Build history of the part. All positions in model axes, mm. A direction names the side the tool comes from. Give positions to 0.01 mm unless a question says otherwise; leave off trailing zeros. Write each loop counter-clockwise with the first axis right and the second up, starting at its lowest first coordinate (ties: lowest second). Pieces come first, ordered by that corner, then holes. Notation, with made-up numbers: M 17,84 L 58,84 A18 cw 58,96 Z; hole C 50.25,15.5 d7. An arc over 180 degrees is marked long. Return JSON: item names as keys, results as strings. Group by question number.
Q1. Pull direction Z, two halves, no side cores. Call faces 4 (the cylindrical face through (-1.08, 0.02, -4.88)), 5 (the flat face through (1, -5, -3.3)), 6 (the flat face through (2, 10, -5)): +Z half, -Z half, draft (parallel to the pull), parting line (faces both ways), or undercut.
Q2. Band-saw the part on B-B, the plane z = 0. Give the cut face in (x, y).
Q3. Band-saw the part on C-C, the plane y = -1. Give the cut face in (x, z), then the cut area to 3 significant figures.
Q4. Band-saw the part on D-D, the plane y = 3.5. Give the cut face in (x, z).
Q5. Wall check: probe 1 along X at (y, z) = (-7, -2.75); probe 2 along Z at (x, y) = (-1.25, 2.5); probe 3 along X at (y, z) = (5.25, -3.25). Give the ranges that are in metal, low to high.
Q6. Band-saw the part on A-A, the plane x = 0. Give the cut face in (y, z).
Q7. Flat gauge pins, fed straight in: pin 1 Ø2 at (x, y) = (-3.5, 2) entering from -Z; pin 2 Ø4 at (y, z) = (-4, 1.5) entering from +X; pin 3 Ø3 at (x, y) = (-1.5, -4.5) entering from +Z. Where does each tip first touch, or does it go through?
Q8. Tool access for faces 1 (the flat face through (-3.3, 5, -1)), 2 (the cylindrical face through (-1.08, -7.54, -4.88)), 3 (the conical face through (5.276, 3.921, -2.188)): list every direction of +Z, -Z, +X, -X, +Y, -Y with a clear straight run to the whole face (end or side of a thin tool).
from build123d import *

# Parameters (mm, degrees)
F0_W           = 5
F0_H           = 3
F3_D           = 6.5
F3_CBORE_D     = 10
F3_CBORE_DEPTH = 5
F4_R           = 5
F4_R_2         = 3.25
F5_DEPTH       = 5


with BuildPart() as f1:
    # F0 (on Top) → F1 (revolve)
    with BuildSketch(Plane.XY):
        Polygon((0, 1.5), (5, 1.5), (7.5, 10), (0, 10), align=None)
        Polygon((0, -10), (7.5, -10), (5, -1.5), (0, -1.5), align=None)
        with Locations((2.5, 0)):
            Rectangle(F0_W, F0_H)
    revolve(axis=Axis((0, 0, 0), (0, -1, 0)))

    # F3 (through all)
    with Locations(Plane(origin=(0, 10, 0), x_dir=(-1, 0, 0), z_dir=(0, 1, 0))):
        with Locations((0, 0)):
            CounterBoreHole(F3_D / 2, F3_CBORE_D / 2, F3_CBORE_DEPTH)

    # F4 (on face) → F5 (cut)
    with BuildSketch(Plane.XZ.offset(10)):
        Circle(F4_R)
        Circle(F4_R_2, mode=Mode.SUBTRACT)
    extrude(amount=-F5_DEPTH, mode=Mode.SUBTRACT)


solid = f1.part
From the geometry:
{
 "1": {"face 4": "parting line", "face 5": "undercut", "face 6": "draft"},
 "2": {"outline": "M -7.5,-10 L -5,-10 L -5,-5 L -3.25,-5 L -3.25,5 L -5,5 L -5,10 L -7.5,10 L -5,1.5 L -5,-1.5 Z; M 3.25,-5 L 5,-5 L 5,-10 L 7.5,-10 L 5,-1.5 L 5,1.5 L 7.5,10 L 5,10 L 5,5 L 3.25,5 Z"},
 "3": {"outline": "C 0,0 d10; hole C 0,0 d6.5", "area": "45.4 mm^2"},
 "4": {"outline": "C 0,0 d11.18; hole C 0,0 d6.5"},
 "5": {"probe 1": "x = -6.02 to -4.18, 4.18 to 6.02", "probe 2": "z = -5.14 to -3, 3 to 5.14", "probe 3": "x = -5.17 to -3.8, 3.8 to 5.17"},
 "6": {"outline": "M -10,-7.5 L -1.5,-5 L 1.5,-5 L 10,-7.5 L 10,-5 L 5,-5 L 5,-3.25 L -5,-3.25 L -5,-5 L -10,-5 Z; M -10,5 L -5,5 L -5,3.25 L 5,3.25 L 5,5 L 10,5 L 10,7.5 L 1.5,5 L -1.5,5 L -10,7.5 Z"},
 "7": {"pin 1": "stops at z = -4.59", "pin 2": "stops at x = 6.24", "pin 3": "stops at z = 6.22"},
 "8": {"face 1": "+Y", "face 2": "-Y", "face 3": "none"}
}
